Build history of the part. All positions in model axes, mm. Face numbers are marked on the shaded views. A direction names the side the tool comes from. Give positions to 0.01 mm unless a question says otherwise; leave off trailing zeros. Write each loop counter-clockwise with the first axis right and the second up, starting at its lowest first coordinate (ties: lowest second). Pieces come first, ordered by that corner, then holes. Notation, with made-up numbers: (86, 16.25) - (128, 16.25) arc R24 ccw to (128, 45.25) - close; hole circle Ø1 at (-30, -11.75). An arc over 180 degrees is marked (long way). Use one line per item in the form item = value. Start each with the question number.
from build123d import *

# Parameters (mm, degrees)
RESSALTO_EXTRUS_O1_DEPTH = 110
ESBO_O2_R                = 10
RESSALTO_EXTRUS_O2_DEPTH = 88.5
ESBO_O3_R                = 10
RESSALTO_EXTRUS_O3_DEPTH = 50
ESBO_O5_W                = 8
ESBO_O5_H                = 8
CORTE_EXTRUS_O1_DEPTH    = 30


with BuildPart() as part:
    # Esboço1 → Ressalto-extrusão1 (new body)
    with BuildSketch(Plane.XY):
        Polygon((-15, 8.660254038), (-15, -8.660254038), (0, -17.320508076), (15, -8.660254038), (15, 8.660254038), (0, 17.320508076), align=None)
    extrude(amount=RESSALTO_EXTRUS_O1_DEPTH)

    # Esboço2 → Ressalto-extrusão2 (add)
    with BuildSketch(Plane.XY.offset(110)):
        Circle(ESBO_O2_R)
    extrude(amount=RESSALTO_EXTRUS_O2_DEPTH)

    # Esboço3 → Ressalto-extrusão3 (add)
    with BuildSketch(Plane(origin=(0, 0, 0), x_dir=(-1, 0, 0), z_dir=(0, 0, -1))):
        Circle(ESBO_O3_R)
    extrude(amount=RESSALTO_EXTRUS_O3_DEPTH)

    # Esboço5 → Corte-extrusão1 (cut)
    with BuildSketch(Plane.XY.offset(198.5)):
        with Locations((0, 10)):
            Rectangle(ESBO_O5_W, ESBO_O5_H)
    extrude(amount=-CORTE_EXTRUS_O1_DEPTH, mode=Mode.SUBTRACT)


solid = part.part
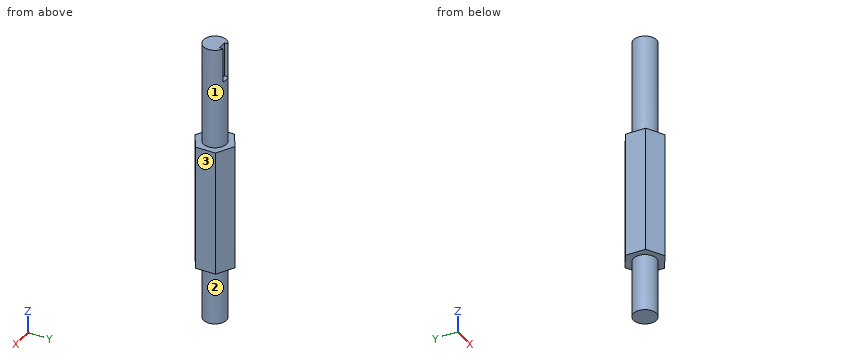
(1) Cut at B-B, the plane z = 123.5. Give the cut face in (x, y).
(2) Pin check, flat tips, straight feed: pin 1 Ø1.2 at (x, y) = (1.5, 7.5) entering from +Z; pin 2 Ø10 at (x, y) = (-2.5, -13.5) entering from +Z; pin 3 Ø2.5 at (y, z) = (7.5, 189.5) entering from -X; pin 4 Ø10 at (y, z) = (-2.5, 136.5) entering from +X. Stop position of each tip, or through.
(3) Cut at D-D, the plane z = 98. Give the cut face in (x, y), then the cut area to 3 significant figures.
(4) Which spindle directions (+Z, -Z, +X, -X, +Y, -Y) get a long thin tool onto all of the face, cutting with end or side? Do the marked faces 1, 2 and 3. Say none if no direction does.
(5) Wall check: line 1 (Y direction, x = 0.75, z = -19.5); line 2 (Z direction, x = -5, y = -11.5); line 3 (Y direction, x = -7.75, z = 179.5). Give the ranges that are in metal, low to high. Write a range as from..to.
(6) Cut at C-C, the plane x = -7. Give the cut face in (y, z), then the cut area to 3 significant figures.
(7) Cut at A-A, the plane y = 0. Give the cut face in (x, z), then the cut area to 3 significant figures.
Solution:
q1.outline = circle Ø20 at (0, 0)
q2.pin_1 = 168.5
q2.pin_2 = 198.5
q2.pin_3 = -7.81
q2.pin_4 = 10
q3.outline = (-15, -8.66) - (0, -17.32) - (15, -8.66) - (15, 8.66) - (0, 17.32) - (-15, 8.66) - close
q3.area = 779 mm2
q4.face_1 = +Z
q4.face_2 = -Z
q4.face_3 = +Z, -Z, +X, +Y, -Y
q5.line_1 = -9.97..9.97
q5.line_2 = 0..110
q5.line_3 = -6.32..6.32
q6.outline = (-13.28, 0) - (-7.14, 0) - (-7.14, -50) - (7.14, -50) - (7.14, 0) - (13.28, 0) - (13.28, 110) - (7.14, 110) - (7.14, 198.5) - (-7.14, 198.5) - (-7.14, 110) - (-13.28, 110) - close
q6.area = 4,900 mm2
q7.outline = (-15, 0) - (-10, 0) - (-10, -50) - (10, -50) - (10, 0) - (15, 0) - (15, 110) - (10, 110) - (10, 198.5) - (-10, 198.5) - (-10, 110) - (-15, 110) - close
q7.area = 6,070 mm2
